The figure shows three views and two pictorial views of one solid part (mm, origin at its lowest corner). Answer the questions. Give positions to 0.01 mm unless a question says otherwise; leave off trailing zeros. Order: outer loops, then holes, each group sorted by start corner. A loop starts at its lowest first (then second) coordinate and runs counter-clockwise, first axis right, second up. Notation, with made-up numbers: (-14.5, -32) - (27.5, -32) arc R25 ccw to (27.5, -16) - close; hole circle Ø7 at (0.25, 6). An arc over 180 degrees is marked (long way). Use a Markdown table: item, result. Add a question column.
1. A cutting plane is placed at B-B on x = 67.5. Determine the outline of the cut face in (y, z).
2. A cutting plane is placed at A-A on z = 2. State how many separate pieces and enclosed holes the cut face has, and give its area (3 significant figures).
3. Consider L1, parallel to Y at x = 32.5, z = 2; L2, parallel to X at y = 7, z = 9; L3, parallel to X at y = 3.5, z = 5. Determine where each line is inside the solid, lowest interval first.
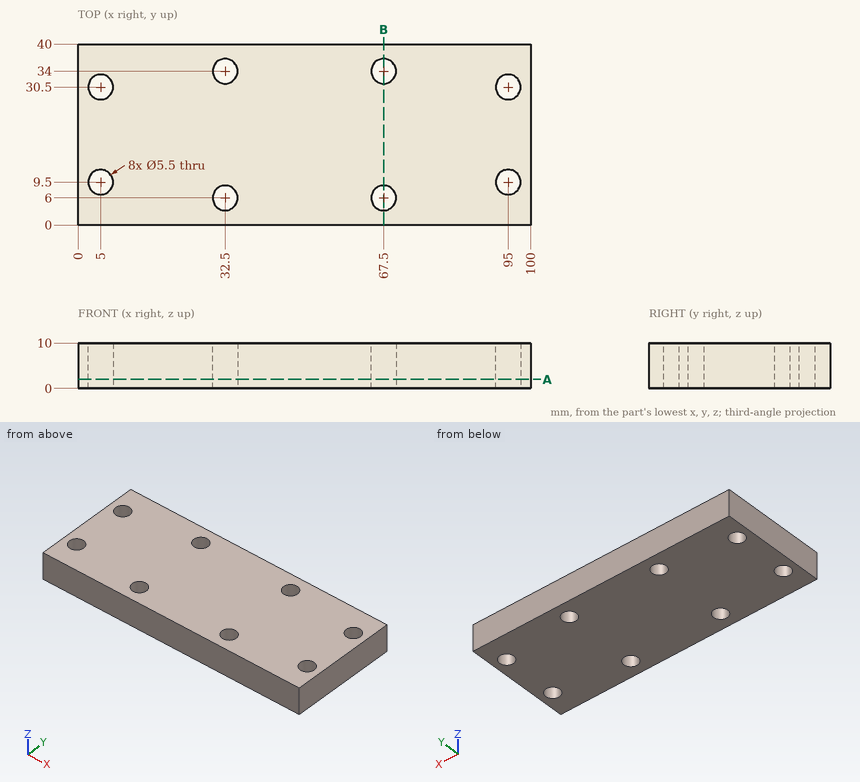
Output values:
| question | item | result |
|---|---|---|
| 1 | outline | (0, 0) - (3.25, 0) - (3.25, 10) - (0, 10) - close; (8.75, 0) - (31.25, 0) - (31.25, 10) - (8.75, 10) - close; (36.75, 0) - (40, 0) - (40, 10) - (36.75, 10) - close |
| 2 | separate pieces | 1 |
| 2 | enclosed holes | 8 |
| 2 | area | 3,810 mm² |
| 3 | L1 | 0 to 3.25, 8.75 to 31.25, 36.75 to 40 |
| 3 | L2 | 0 to 3.85, 6.15 to 29.94, 35.06 to 64.94, 70.06 to 93.85, 96.15 to 100 |
| 3 | L3 | 0 to 31.35, 33.65 to 66.35, 68.65 to 100 |
